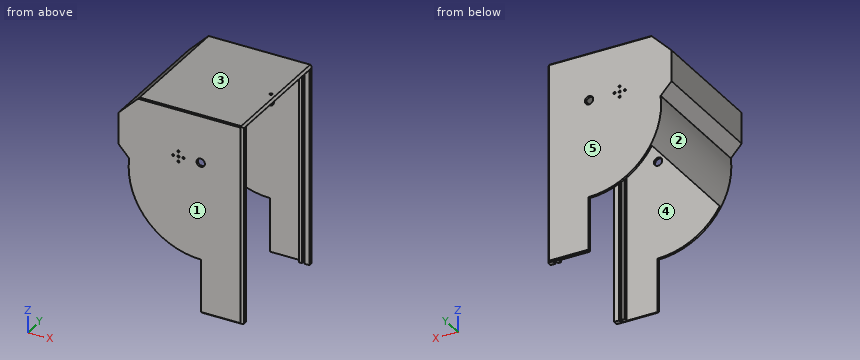
Autodesk Fusion 360 part; units mm, degrees
sketch "Sketch1" plane through (0, 0, 0) normal (0, 1, 0) x (1, 0, 0)
  line L0 (20, -60) -> (120, -60)
  line L1 (120, -60) -> (120, 0)
  line L2 (0, -10) -> (0, -40)
  line L3 (10.4331, 1.3041) -> (10.5405, 1.3176)
  line L4 (80, 80) -> (80, 132)
  line L5 (80, 132) -> (120, 132)
  line L6 (120, 132) -> (120, 0)
  line L7 (0, -40) -> (20, -60)
  line L8 (0, -10) -> (10.4331, 1.3041)
  arc A0 (80, 80) -> (10.5405, 1.3176) centre (80, 10) ccw
  dimension "d2" = 60
  dimension "d3" = 132
  dimension "d6" = 15.3829
  dimension "d7" = 30
  dimension "d8" = 28.2843
  dimension "d9" = 100
  dimension "d10" = 40
  dimension "d48" = 70
extrude "Extrude1" add sketch "Sketch1" along normal blind 120.4
sketch "Sketch3" plane through (120, 0, 0) normal (1, 0, 0) x (0, 1, 0)
  line L0 (0, 60) -> (0, -132)
  line L1 (0, -132) -> (120.4, -132)
  line L2 (120.4, -132) -> (120.4, 60)
  line L3 (120.4, 60) -> (0, 60)
  line L4 (2.1, 57.9) -> (118.3, 57.9)
  line L5 (118.3, 57.9) -> (118.3, -56)
  line L6 (2.1, -56) -> (2.1, 57.9)
  line L7 (2.1, -56) -> (2.1, -132)
  line L8 (118.3, -132) -> (118.3, -56)
  dimension "d14" = 2.1
  dimension "d15" = 2.1
  dimension "d16" = 2.1
  dimension "d19" = 2.1
  dimension "d20" = 2.1
extrude "Extrude2" cut sketch "Sketch3" against normal blind 100 contours L1 L4 L5 L6 L7 L8
sketch "Sketch5" plane through (0, 0, 57.9) normal (0, 0, -1) x (1, 0, 0)
  line L0 (120, -118.3) -> (120, -2.1)
  line L1 (20, -2.1) -> (20, -118.3)
  line L2 (20, -118.3) -> (120, -118.3)
  line L3 (120, -118.3) -> (112.8, -118.3)
  line L4 (112.8, -118.3) -> (112.8, -2.1)
  line L5 (112.8, -2.1) -> (120, -2.1)
  line L6 (120, -2.1) -> (120, -118.3)
  line L7 (120, -2.1) -> (20, -2.1)
  dimension "d24" = 7.2
extrude "Extrude3" cut sketch "Sketch5" against normal blind 2.5 contours L0 L2 L3 L4 L5 L6 L7
sketch "Sketch7" plane through (0, 2.1, 0) normal (0, 1, 0) x (-1, 0, 0)
  line L0 (-80, -132) -> (-80, -80)
  line L1 (-20, -46.0555) -> (-20, 57.9)
  line L2 (-20, 57.9) -> (-112.8, 57.9)
  line L3 (-112.8, 57.9) -> (-112.8, 60)
  line L4 (-112.8, 60) -> (-120, 60)
  line L5 (-120, 60) -> (-120, -132)
  line L6 (-120, -132) -> (-80, -132)
  line L7 (-112, 57.9) -> (-120, 57.9)
  line L8 (-120, 57.9) -> (-120, -132)
  line L9 (-120, -132) -> (-112, -132)
  line L10 (-112, -132) -> (-112, 57.9)
  arc A0 (-80, -80) -> (-20, -46.0555) centre (-80, -10) ccw
  dimension "d27" = 8
extrude "Extrude4" add sketch "Sketch7" along normal blind 3.6 contours L2 L5 L6 L7 L8 L9 L10
sketch "Sketch8" plane through (0, 0, 57.9) normal (0, 0, 1) x (-1, 0, 0)
  line L0 (-112.8, -5.7) -> (-112.8, -2.1)
  line L1 (-112.8, -2.1) -> (-120, -2.1)
  line L2 (-120, -2.1) -> (-120, -5.7)
  line L3 (-120, -5.7) -> (-112.8, -5.7)
  line L4 (-112.8, -2.1) -> (-115.3, -2.1)
  line L5 (-115.3, -2.1) -> (-115.3, -5.7)
  line L6 (-115.3, -5.7) -> (-112.8, -5.7)
  line L7 (-112.8, -5.7) -> (-112.8, -2.1)
  dimension "d30" = 2.5
extrude "Extrude5" cut sketch "Sketch8" against normal blind 190 contours L0 L1 L3 L4 L5 L6 L7
sketch "Sketch9" plane through (0, 118.3, 0) normal (0, -1, 0) x (1, 0, 0)
  line L0 (80, -80) -> (80, -132)
  line L1 (80, -132) -> (120, -132)
  line L2 (120, -132) -> (120, 60)
  line L3 (120, 60) -> (112.8, 60)
  line L4 (112.8, 60) -> (112.8, 57.9)
  line L5 (112.8, 57.9) -> (20, 57.9)
  line L6 (20, 57.9) -> (20, -46.0555)
  line L7 (112, 57.9) -> (120, 57.9)
  line L8 (120, 57.9) -> (120, -132)
  line L9 (120, -132) -> (112, -132)
  line L10 (112, -132) -> (112, 57.9)
  arc A0 (20, -46.0555) -> (80, -80) centre (80, -10) ccw
  dimension "d33" = 8
extrude "Extrude6" add sketch "Sketch9" along normal blind 3.6 contours L1 L2 L5 L7 L8 L9 L10
sketch "Sketch10" plane through (0, 0, 57.9) normal (0, 0, 1) x (-1, 0, 0)
  line L0 (-112.8, -118.3) -> (-112.8, -114.7)
  line L1 (-112.8, -114.7) -> (-120, -114.7)
  line L2 (-120, -114.7) -> (-120, -118.3)
  line L3 (-120, -118.3) -> (-112.8, -118.3)
  line L4 (-112.8, -118.3) -> (-115.3, -118.3)
  line L5 (-115.3, -118.3) -> (-115.3, -114.7)
  line L6 (-115.3, -114.7) -> (-112.8, -114.7)
  line L7 (-112.8, -114.7) -> (-112.8, -118.3)
  dimension "d36" = 2.5
extrude "Extrude7" cut sketch "Sketch10" against normal blind 190 contours L0 L1 L3 L4 L5 L6 L7
chamfer "Chamfer1" distance 1 angle 45 4 edges at (100, 0, -132) (100, 120.4, -132) (70, 0, 60) (70, 120.4, 60)
sketch "Sketch15" plane through (112.8, 0, 0) normal (1, 0, 0) x (0, 1, 0)
  line L0 (118.3, 60) -> (2.1, 60)
  line L1 (2.1, 60) -> (2.1, -132)
  line L2 (5.7, -132) -> (5.7, 57.9)
  line L3 (5.7, 57.9) -> (114.7, 57.9)
  line L4 (114.7, 57.9) -> (114.7, -132)
  line L5 (118.3, -132) -> (118.3, 60)
  line L6 (2.1, 60) -> (118.3, 60)
  line L7 (118.3, 60) -> (118.3, 57.9)
  line L8 (118.3, 57.9) -> (2.1, 57.9)
  line L9 (2.1, 57.9) -> (2.1, 60)
  line L10 (2.1, -132) -> (5.7, -132)
  line L11 (114.7, -132) -> (118.3, -132)
extrude "Extrude11" add sketch "Sketch15" along normal blind 7.2 contours L0 L1 L3 L5 L6 L7 L8 L9
sketch "Sketch16" plane through (0, 2.1, 0) normal (0, 1, 0) x (-1, 0, 0)
  line L0 (-112, 57.9) -> (-112, -132)
  line L1 (-112, -132) -> (-80, -132)
  line L2 (-80, -132) -> (-80, -80)
  arc A0 (-80, -80) -> (-20, -46.0555) centre (-80, -10) ccw
  line L3 (-20, -46.0555) -> (-20, 57.9)
  line L4 (-20, 57.9) -> (-112, 57.9)
  line L5 (-112, 57.9) -> (-110, 57.9)
  line L6 (-110, 57.9) -> (-110, -132)
  line L7 (-110, -132) -> (-112, -132)
  line L8 (-112, -132) -> (-112, 57.9)
  dimension "d54" = 2
extrude "Extrude12" add sketch "Sketch16" along normal blind 3.6 contours L0 L1 L4 L5 L6 L7 L8
sketch "Sketch17" plane through (0, 118.3, 0) normal (0, -1, 0) x (1, 0, 0)
  line L0 (112, -132) -> (112, 57.9)
  line L1 (112, 57.9) -> (20, 57.9)
  line L2 (20, 57.9) -> (20, -46.0555)
  arc A0 (20, -46.0555) -> (80, -80) centre (80, -10) ccw
  line L3 (80, -80) -> (80, -132)
  line L4 (80, -132) -> (112, -132)
  line L5 (112, 57.9) -> (110, 57.9)
  line L6 (110, 57.9) -> (110, -132)
  line L7 (110, -132) -> (112, -132)
  line L8 (112, -132) -> (112, 57.9)
  dimension "d57" = 2
extrude "Extrude13" add sketch "Sketch17" along normal blind 3.6 contours L0 L1 L4 L5 L6 L7 L8
sketch "Sketch18" plane through (0, 0, 57.9) normal (0, 0, -1) x (1, 0, 0)
  line L0 (110, -118.3) -> (110, -114.7)
  line L1 (110, -114.7) -> (112.8, -114.7)
  line L2 (112.8, -114.7) -> (112.8, -118.3)
  line L3 (112.8, -118.3) -> (115.3, -118.3)
  line L4 (115.3, -118.3) -> (115.3, -114.7)
  line L5 (115.3, -114.7) -> (120, -114.7)
  line L6 (120, -114.7) -> (120, -5.7)
  line L7 (120, -5.7) -> (115.3, -5.7)
  line L8 (115.3, -5.7) -> (115.3, -2.1)
  line L9 (115.3, -2.1) -> (112.8, -2.1)
  line L10 (112.8, -2.1) -> (112.8, -5.7)
  line L11 (112.8, -5.7) -> (110, -5.7)
  line L12 (110, -5.7) -> (110, -2.1)
  line L13 (110, -2.1) -> (20, -2.1)
  line L14 (20, -2.1) -> (20, -118.3)
  line L15 (20, -118.3) -> (110, -118.3)
  circle A0 centre (25, -84.8) radius 2.5
  circle A1 centre (25, -35.8) radius 2.5
  circle A2 centre (83, -35.8) radius 2.5
  circle A3 centre (83, -84.8) radius 2.5
  circle A4 centre (83, -35.8) radius 1.375
  circle A5 centre (25, -35.8) radius 1.375
  circle A6 centre (83, -84.8) radius 1.375
  circle A7 centre (25, -84.8) radius 1.375
  dimension "d60" = 5
  dimension "d61" = 5
  dimension "d62" = 49
  dimension "d63" = 49
  dimension "d64" = 58
  dimension "d65" = 33.5
  dimension "d66" = 33.5
  dimension "d67" = 5
  dimension "d68" = 5
  dimension "d71" = 2.75
  dimension "d72" = 2.75
  dimension "d73" = 2.75
  dimension "d74" = 2.75
  dimension "d77" = 5
  dimension "d78" = 58
  dimension "d79" = 5
extrude "Extrude15" add sketch "Sketch18" along normal blind 5 contours A0 | A1 | A2 | A3
chamfer "Chamfer2" distance 2 angle 45 3 edges at (120, 60.2, 60) (120, 0, -36) (120, 120.4, -36)
sketch "Sketch19" plane through (0, 120.4, 0) normal (0, 1, 0) x (-1, 0, 0)
  line L0 (-118, 59) -> (-118, -131)
  line L1 (-118, -131) -> (-80, -131)
  line L2 (-80, -131) -> (-80, -80)
  arc A0 (-80, -80) -> (-10.5405, -1.3176) centre (-80, -10) ccw
  line L3 (-10.5405, -1.3176) -> (-10.4331, -1.3041)
  line L4 (-10.4331, -1.3041) -> (0, 10)
  line L5 (0, 10) -> (0, 40)
  line L6 (0, 40) -> (-19, 59)
  line L7 (-19, 59) -> (-118, 59)
  circle A1 centre (-50, 14) radius 1
  circle A2 centre (-50, 19) radius 1
  circle A3 centre (-45, 14) radius 1
  circle A4 centre (-55, 14) radius 1
  circle A5 centre (-50, 9) radius 1
  line L8 (-110, 57.9) -> (-110, -132)
  dimension "d81" = 2
  dimension "d82" = 2
  dimension "d83" = 2
  dimension "d84" = 2
  dimension "d85" = 2
  dimension "d86" = 5
  dimension "d87" = 5
  dimension "d88" = 5
  dimension "d89" = 5
  dimension "d90" = 60
  dimension "d93" = 45
extrude "Extrude16" cut sketch "Sketch19" against normal blind 5 contours A1 | A2 | A3 | A4 | A5
sketch "Sketch20" plane through (0, 0, 0) normal (0, -1, 0) x (1, 0, 0)
  line L0 (118, -131) -> (118, 59)
  line L1 (118, 59) -> (19, 59)
  line L2 (19, 59) -> (0, 40)
  line L3 (0, 40) -> (0, 10)
  line L4 (0, 10) -> (10.4331, -1.3041)
  line L5 (10.4331, -1.3041) -> (10.5405, -1.3176)
  arc A0 (10.5405, -1.3176) -> (80, -80) centre (80, -10) ccw
  line L6 (80, -80) -> (80, -131)
  line L7 (80, -131) -> (118, -131)
  circle A1 centre (58, 14) radius 1
  circle A2 centre (58, 19) radius 1
  circle A3 centre (63, 14) radius 1
  circle A4 centre (53, 14) radius 1
  circle A5 centre (58, 9) radius 1
  dimension "d94" = 2
  dimension "d95" = 2
  dimension "d96" = 2
  dimension "d97" = 2
  dimension "d98" = 2
  dimension "d99" = 5
  dimension "d100" = 5
  dimension "d101" = 5
  dimension "d102" = 5
  dimension "d103" = 60
  dimension "d104" = 45
extrude "Extrude17" cut sketch "Sketch20" against normal blind 5 contours A1 | A2 | A3 | A4 | A5
sketch "Sketch21" plane through (0, 0, 0) normal (0, -1, 0) x (1, 0, 0)
  circle A0 centre (58, 9) radius 1
  circle A1 centre (63, 14) radius 1
  circle A2 centre (53, 14) radius 1
  circle A3 centre (58, 19) radius 1
  circle A4 centre (58, 14) radius 1
  line L0 (118, -131) -> (118, 59)
  line L1 (118, 59) -> (19, 59)
  line L2 (19, 59) -> (0, 40)
  line L3 (0, 40) -> (0, 10)
  line L4 (0, 10) -> (10.4331, -1.3041)
  line L5 (10.4331, -1.3041) -> (10.5405, -1.3176)
  arc A5 (10.5405, -1.3176) -> (80, -80) centre (80, -10) ccw
  line L6 (80, -80) -> (80, -131)
  line L7 (80, -131) -> (118, -131)
  circle A6 centre (79.5207, 14) radius 4.025
  dimension "d107" = 8.05
extrude "Extrude18" cut sketch "Sketch21" against normal blind 170 contours A6
sketch "Sketch22" plane through (0, 0, 60) normal (0, 0, 1) x (-1, 0, 0)
  line L0 (-118, -1) -> (-118, -119.4)
  line L1 (-118, -119.4) -> (-20, -119.4)
  line L2 (-20, -119.4) -> (-20, -1)
  line L3 (-20, -1) -> (-118, -1)
  circle A0 centre (-113.6, -60.2) radius 1.375
  dimension "d110" = 4.4
  dimension "d111" = 2.75
  dimension "d112" = 59.2
extrude "Extrude19" cut sketch "Sketch22" against normal blind 3 contours A0
Input: part model. Units: mm. Frame: model coordinates. Face numbers are marked on the shaded views. A direction names the side the tool comes from. Give positions to 0.01 mm unless a question says otherwise; leave off trailing zeros. Loops run counter-clockwise (first coordinate to the right, second up) from the corner with the lowest first, then second, coordinate; pieces in that order, holes last. Notation, with made-up numbers: (-8, -38.75) -> (29, -38.75) arc R33 ccw to (29, -10.75) -> close; hole circle Ø1 at (30.5, 59.25). An arc over 180 degrees is marked (long way). Answer as a JSON object with one key per item and string values. Group by question number.
Item 1: Line query: probe 1 along Y at (x, z) = (25, 56) (3 decimals); probe 2 along Y at (x, z) = (66, -55.5); probe 3 along Z at (x, y) = (50, 118.9). Output: solid intervals per line, ascending.
Item 2: Pin query (flat end, axial travel): P1, Ø1.1, axis at y = 4, z = -12, coming from the -X side (3 decimals); P2, Ø8, axis at x = 59, y = 13.5, coming from the -Z side; P3, Ø2, axis at y = 56, z = -48, coming from the +X side; P4, Ø5.5, axis at x = 24.5, y = 83.5, coming from the -Z side. Return the tip coordinate at first contact, or that it passes through.
Item 3: Pull-direction query (Z, two-part tool) for the marked faces 1, 2 and 3; classes: released by +Z, released by -Z, zero draft, split by the parting line, or undercut.
Item 4: Cut plane A-A, the plane z = -99.5. Return the cut outline in (x, y).
Item 5: Reachability of the marked faces 4 and 5 from +Z, -Z, +X, -X, +Y, -Y: full face, straight path, thin tool, end or side. Return the list, or none.
Item 6: Cut plane C-C, the plane z = 44. Return the cut outline in (x, y), and give its area (3 significant figures).
Item 7: Cut plane B-B, the plane y = 15. Return the cut outline in (x, z), and give its area (3 significant figures).
Item 8: Cut plane D-D, the plane z = -18. Return the cut outline in (x, y).
Checks:
{
 "1": {"probe 1": "y = 0 to 2.1, 33.3 to 34.425, 37.175 to 38.3, 82.3 to 83.425, 86.175 to 87.3, 118.3 to 120.4", "probe 2": "y = 0 to 2.1, 118.3 to 120.4", "probe 3": "z = -73.25 to 8, 10 to 13, 15 to 18, 20 to 60"},
 "2": {"P1": "stops at x = 10.015", "P2": "stops at z = 57.9", "P3": "passes through", "P4": "stops at z = 52.9"},
 "3": {"face 1": "zero draft", "face 2": "undercut", "face 3": "released by +Z"},
 "4": {"outline": "(80, 0) -> (118, 0) -> (120, 2) -> (120, 5.7) -> (115.3, 5.7) -> (115.3, 2.1) -> (112.8, 2.1) -> (112.8, 5.7) -> (110, 5.7) -> (110, 2.1) -> (80, 2.1) -> close; (80, 118.3) -> (110, 118.3) -> (110, 114.7) -> (112.8, 114.7) -> (112.8, 118.3) -> (115.3, 118.3) -> (115.3, 114.7) -> (120, 114.7) -> (120, 118.4) -> (118, 120.4) -> (80, 120.4) -> close"},
 "5": {"face 4": "-Z", "face 5": "+Z, -Z, +X, -X, +Y"},
 "6": {"outline": "(4, 0) -> (118, 0) -> (120, 2) -> (120, 5.7) -> (115.3, 5.7) -> (115.3, 2.1) -> (112.8, 2.1) -> (112.8, 5.7) -> (110, 5.7) -> (110, 2.1) -> (20, 2.1) -> (20, 118.3) -> (110, 118.3) -> (110, 114.7) -> (112.8, 114.7) -> (112.8, 118.3) -> (115.3, 118.3) -> (115.3, 114.7) -> (120, 114.7) -> (120, 118.4) -> (118, 120.4) -> (4, 120.4) -> close", "area": "2,400 mm²"},
 "7": {"outline": "(0, 10) -> (10.43, -1.3) -> (10.54, -1.32) arc R70 ccw to (20, -46.06) -> (20, 57.9) -> (120, 57.9) -> (120, 58) -> (118, 60) -> (20, 60) -> (0, 40) -> close", "area": "1,500 mm²"},
 "8": {"outline": "(10.46, 0) -> (118, 0) -> (120, 2) -> (120, 5.7) -> (115.3, 5.7) -> (115.3, 2.1) -> (112.8, 2.1) -> (112.8, 5.7) -> (110, 5.7) -> (110, 2.1) -> (20, 2.1) -> (20, 118.3) -> (110, 118.3) -> (110, 114.7) -> (112.8, 114.7) -> (112.8, 118.3) -> (115.3, 118.3) -> (115.3, 114.7) -> (120, 114.7) -> (120, 118.4) -> (118, 120.4) -> (10.46, 120.4) -> close"}
}
